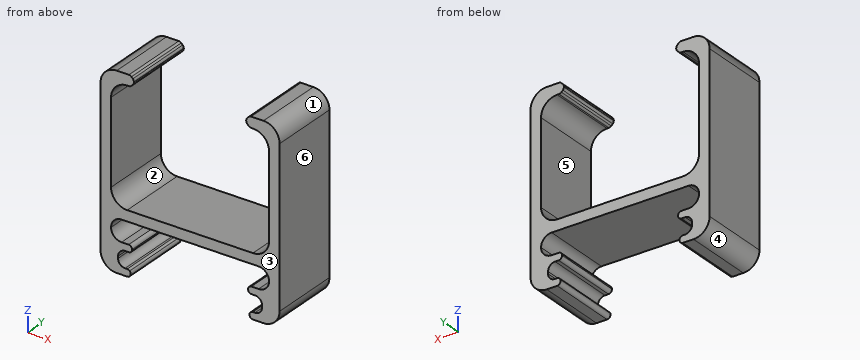
Autodesk Fusion 360 part; units mm, degrees
sketch "Sketch1" plane through (0, 0, 0) normal (0, 1, 0) x (1, 0, 0)
  line L0 (-8.25, 14.8) -> (-12.75, 14.8)
  line L1 (-12.75, 14.8) -> (-8.25, 14.8)
  line L2 (-8.25, 13.8) -> (-10.25, 13.8)
  line L3 (-11.25, -10.5) -> (-8, -10.5)
  line L4 (-8, -10.5) -> (-8, -12)
  line L5 (-8, -12) -> (-12.75, -12)
  line L6 (-8.25, 13.8) -> (-8.25, 14.8)
  line L7 (-10.25, 13.8) -> (-10.25, 11.5)
  line L8 (-10.25, 11.5) -> (-8.25, 11.5)
  line L9 (-8.25, 11.5) -> (-8.25, 10.5)
  line L10 (-8.25, 10.5) -> (-11.25, 10.5)
  line L11 (-12.75, 14.8) -> (-12.75, -12)
  line L12 (0, 7.5) -> (-11.25, 7.5)
  line L13 (-11.25, 7.5) -> (-11.25, 10.5)
  line L14 (0, 7.5) -> (0, 6)
  line L15 (0, 6) -> (-11.25, 6)
  line L16 (-11.25, 6) -> (-11.25, -10.5)
  dimension "d1" = 2.3
  dimension "d2" = 1
  dimension "d3" = 1
  dimension "d5" = 2
  dimension "d8" = 1.5
  dimension "d11" = 8
  dimension "d13" = 10.5
  dimension "d14" = 10.5
  dimension "d17" = 1
  dimension "d28" = 1.5
  dimension "d29" = 1.5
  dimension "d30" = 3
  dimension "d34" = 10.25
extrude "Extrude1" add sketch "Sketch1" along normal blind 10 makes body 1
chamfer "Chamfer1" distance 0.5 angle 45 3 edges at (-8.25, 5, -13.8) (-8, 5, 12) (-8, 5, 10.5) on bodies 1
fillet "Fillet1" radius 0.5 6 edges at (-8, 5, 11.5) (-8, 5, 11) (-8.5, 5, 12) (-8.5, 5, 10.5) (-8.25, 5, -14.3) (-8.75, 5, -13.8) on bodies 1
fillet "Fillet2" radius 2.3 4 edges at (-12.75, 5, 12) (-12.75, 5, -14.8) (-11.25, 5, -6) (-11.25, 5, 10.5) on bodies 1
fillet "Fillet3" radius 0.5 3 edges at (-8.25, 5, -14.8) (-8.25, 5, -11.5) (-8.25, 5, -10.5) on bodies 1
fillet "Fillet4" radius 1 2 edges at (-10.25, 5, -13.8) (-10.25, 5, -11.5) on bodies 1
fillet "Fillet5" radius 1.5 2 edges at (-11.25, 5, -10.5) (-11.25, 5, -7.5) on bodies 1
mirror "Mirror1" about plane through (0, 0, -7.5) normal (1, 0, 0) of bodies 1 makes body 2
combine "Combine1" operation add target body 1 tool bodies 2
Source: CAD feature listing. Evaluate the final solid. Frame: model axes, mm. Face numbers are marked on the shaded views. A direction names the side the tool comes from. Round coordinates to 2 decimals unless told otherwise and drop trailing zeros. Order: outer loops, then holes, each group sorted by start corner. A loop starts at its lowest first (then second) coordinate and runs counter-clockwise, first axis right, second up. Notation, with made-up numbers: (-25, 42.5) -> (-8, 42.5) arc R6 cw to (-8, 47.5) -> close; hole circle Ø10 at (23, -10.5). An arc over 180 degrees is marked (long way). Answer as CSV lines item,"result".
Item 1: Section A-A, the plane z = 1. Return loops of the section in (x, y), plus the area to 3 significant figures.
A:
outline,"(-12.75, 0) -> (-11.25, 0) -> (-11.25, 10) -> (-12.75, 10) -> close; (11.25, 0) -> (12.75, 0) -> (12.75, 10) -> (11.25, 10) -> close"
area,"30.0 mm²"
Item 2: Pull-direction query (Z, two-part tool) for the marked faces 1, 2, 3 and 4; classes: pulls with the +Z half, pulls with the -Z half, needs draft (parallel to the pull), parting line crosses it, or undercut.
A:
face 1,"pulls with the +Z half"
face 2,"undercut"
face 3,"needs draft"
face 4,"pulls with the -Z half"
Item 3: Line query: L1, parallel to X at y = 2.25, z = -2.25; L2, parallel to Z at x = 8.75, y = 1.5; L3, parallel to Z at x = 1, y = 0.75. Output: solid intervals per line, ascending.
A:
L1,"-12.75 to -11.25, 11.25 to 12.75"
L2,"-14.76 to -13.84, -11.5 to -10.5, -7.5 to -6, 10.5 to 12"
L3,"-7.5 to -6"
Item 4: Reachability of the marked faces 5 and 6 from +Z, -Z, +X, -X, +Y, -Y: full face, straight path, thin tool, end or side. Return the list, or none.
A:
face 5,"+Y, -Y"
face 6,"+Z, -Z, +X, +Y, -Y"
Item 5: Pin query (flat end, axial travel): pin 1 Ø5 at (x, z) = (4, -12) entering from +Y; pin 2 Ø3 at (x, y) = (-0.5, 1) entering from -Z. Return the tip coordinate at first contact, or that it passes through.
A:
pin 1,"through"
pin 2,"z = -7.5"
Item 6: Section B-B, the plane x = -7.25. Return loops of the section in (y, z), plus the area to 3 significant figures.
A:
outline,"(0, -7.5) -> (10, -7.5) -> (10, -6) -> (0, -6) -> close"
area,"15.0 mm²"
